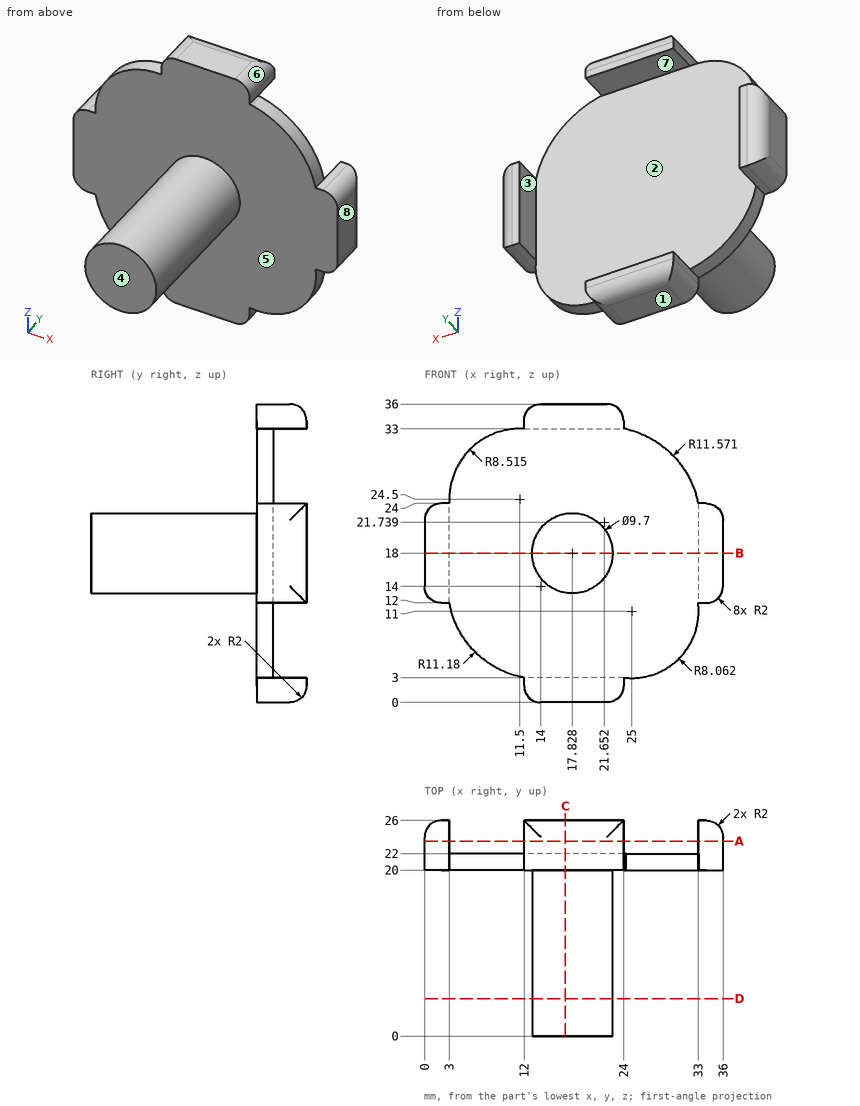
Source: three-view drawing plus pictorial views. Frame: mm from the lowest corner of the part. A direction names the side the tool comes from. Round coordinates to 2 decimals unless told otherwise and drop trailing zeros. Write each loop counter-clockwise with the first axis right and the second up, starting at its lowest first coordinate (ties: lowest second). Pieces come first, ordered by that corner, then holes. Notation, with made-up numbers: M 58.25,-3 L 103.25,-3 A36 cw 103.25,32 Z; hole C 68.25,87.5 d10. An arc over 180 degrees is marked long. Write item = value, one per line.
Item 1: Pull-direction query (Z, two-part tool) for the marked faces 6, 7 and 8; classes: pulls with the +Z half, pulls with the -Z half, needs draft (parallel to the pull), parting line crosses it, or undercut.
Findings:
face_6 = pulls with the +Z half
face_7 = undercut
face_8 = needs draft
Item 2: Pin query (flat end, axial travel): P1, Ø4, axis at y = 21.5, z = 11, coming from the -X side; P2, Ø4.5, axis at y = 24.5, z = 16, coming from the -X side; P3, Ø1.1, axis at x = 2.5, y = 24.5, coming from the -Z side; P4, Ø4, axis at x = 28, z = 21.5, coming from the -Y side. Return the tip coordinate at first contact, or that it passes through.
Findings:
P1 = 0.27
P2 = 0
P3 = 12
P4 = 20
Item 3: Material intervals for line 1 along X through (y, z) = (23.25, 20); line 2 along Y through (x, z) = (28, 17); line 3 along X through (y, z) = (17, 21.5) (1 decimal), sorted ascending. Write a range as [from, to].
Findings:
line_1 = [0, 3], [33, 36]
line_2 = [20, 22]
line_3 = [14.5, 21.2]
Item 4: Section query C-C on x = 17. Return loops of the section in (y, z).
Findings:
outline = M 0,13.22 L 20,13.22 L 20,0 L 24,0 A2 ccw 26,2 L 26,3 L 22,3 L 22,33 L 26,33 L 26,34 A2 ccw 24,36 L 20,36 L 20,22.78 L 0,22.78 Z
Item 5: Section query B-B on z = 18. Return loops of the section in (x, y).
Findings:
outline = M 0,20 L 12.98,20 L 12.98,0 L 22.68,0 L 22.68,20 L 36,20 L 36,24 A2 ccw 34,26 L 33,26 L 33,22 L 3,22 L 3,26 L 2,26 A2 ccw 0,24 Z
Item 6: Section query D-D on y = 4.5. Return loops of the section in (x, z), then the cut area to 3 significant figures.
Findings:
outline = C 17.83,18 d9.7
area = 73.9 mm^2
Item 7: Section query A-A on y = 23.5. Return loops of the section in (x, z), then the cut area to 3 significant figures.
Findings:
outline = M 0,14 A2 ccw 2,12 L 3,12 L 3,24 L 2,24 A2 ccw 0,22 Z; M 12,2 A2 ccw 14,0 L 22,0 A2 ccw 24,2 L 24,3 L 12,3 Z; M 12,33 L 24,33 L 24,34 A2 ccw 22,36 L 14,36 A2 ccw 12,34 Z; M 33,12 L 34,12 A2 ccw 36,14 L 36,22 A2 ccw 34,24 L 33,24 Z
area = 137 mm^2
Item 8: Access query for the marked faces 1, 2, 3, 4 and 5. Directions: +Z, -Z, +X, -X, +Y, -Y. A direction counts if a zero-diameter tool reaches every point of the face in a straight line with its end or side. Return the directions, or none.
Findings:
face_1 = -Z, +X, -X, +Y, -Y
face_2 = +Y
face_3 = +Z, -Z, +Y
face_4 = +Z, -Z, +X, -X, -Y
face_5 = -Y
